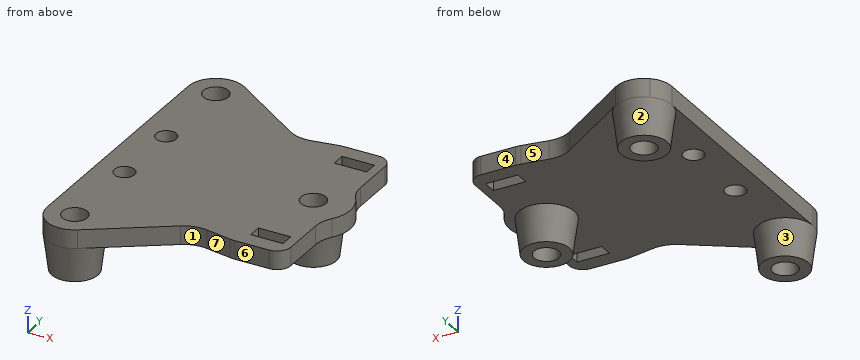
```python
from build123d import *

# Parameters (mm, degrees)
SKETCH_1_R          = 2.2
SKETCH_1_R_2        = 2.7
EXTRUDE_1_DEPTH     = 4
CUT_EXTRUDE_1_REACH = 59.017
EXTRUDE_START       = -4
SKETCH_6_W          = 7
SKETCH_6_H          = 3
SKETCH_6_R          = 2.7
EXTRUDE_3_DEPTH     = 4
FILLET_1_R          = 7
FILLET_2_R          = 3


with BuildPart() as part:
    # 草图1 → 凸台-拉伸1 (new body)
    with BuildSketch(Plane.XY):
        with BuildLine():
            Line((-22.03836949, 31.611607058), (-45, 12.5))
            Line((-45, 12.5), (-45, -12.5))
            Line((-45, -12.5), (-22.03836949, -31.611607058))
            ThreePointArc((-22.03836949, -31.611607058), (-18.500125226, -32.992489036), (-14.841614052, -31.972046241))
            Line((-14.841614052, -31.972046241), (22.677847931, -6.629394988))
            ThreePointArc((22.677847931, -6.629394988), (26.2, 0), (22.677847931, 6.629394988))
            Line((22.677847931, 6.629394988), (-14.841614052, 31.972046241))
            ThreePointArc((-14.841614052, 31.972046241), (-18.500125226, 32.992489036), (-22.03836949, 31.611607058))
        make_face()
        with Locations((-18.2, -8)):
            Circle(SKETCH_1_R, mode=Mode.SUBTRACT)
        with Locations((-18.2, 8)):
            Circle(SKETCH_1_R, mode=Mode.SUBTRACT)
        with Locations((-34.2, 0)):
            Circle(SKETCH_1_R, mode=Mode.SUBTRACT)
        with Locations((-18.2, 27)):
            Circle(SKETCH_1_R_2, mode=Mode.SUBTRACT)
        with Locations((-18.2, -27)):
            Circle(SKETCH_1_R_2, mode=Mode.SUBTRACT)
        with Locations((18.2, 0)):
            Circle(SKETCH_1_R_2, mode=Mode.SUBTRACT)
    extrude(amount=EXTRUDE_1_DEPTH)

    # 草图4 → 旋转1 (revolve)
    with BuildSketch(Plane(origin=(-25.021499827, 16.900859193, 0), x_dir=(0, 0, -1), z_dir=(0.8286743735186554, -0.5597309913462574, 0)), mode=Mode.PRIVATE) as revolve_1_sk:
        Polygon((7.7, 17.187104043), (7.7, 14.887104043), (0, 14.887104043), (0, 18.187104043), align=None)
    revolve_1 = revolve(revolve_1_sk.sketch.rotate(Axis((-18.2, 27, 1000.278995542), (0, 0, -1)), 55.962803956), axis=Axis((-18.2, 27, 1000.278995542), (0, 0, -1)))

    # 镜向1: 旋转1 across plane
    add(revolve_1.mirror(Plane.ZX))

    # 草图5 → 切除-拉伸1 (cut, up to next)
    with BuildSketch(Plane.XY.offset(4), mode=Mode.PRIVATE) as cut_extrude_1_sk1:
        with BuildLine():
            Line((-24.2, -27), (-24.2, 27))
            ThreePointArc((-24.2, 27), (-23.632780915, 29.546545018), (-22.03836949, 31.611607058))
            Line((-22.03836949, 31.611607058), (-45, 12.5))
            Line((-45, 12.5), (-45, -12.5))
            Line((-45, -12.5), (-22.03836949, -31.611607058))
            ThreePointArc((-22.03836949, -31.611607058), (-23.632780915, -29.546545018), (-24.2, -27))
        make_face()
    cut_extrude_1_tool1 = extrude(cut_extrude_1_sk1.sketch, amount=-CUT_EXTRUDE_1_REACH, mode=Mode.PRIVATE) & part.part
    add(cut_extrude_1_tool1.solids().sort_by_distance((-33.15819, 0, 4))[0], mode=Mode.SUBTRACT)

    # 草图6 → 凸台-拉伸3 (add)
    with BuildSketch(Plane.XY.offset(4).offset(EXTRUDE_START)):
        Polygon((12.5, -13.504057816), (3.649903477, -19.481886332), (12.5, -21), (23.5, -21), (23.5, 21), (12.5, 21), (3.649903477, 19.481886332), (12.5, 13.504057816), align=None)
        with Locations((18, -16)):
            Rectangle(SKETCH_6_W, SKETCH_6_H, mode=Mode.SUBTRACT)
        with Locations((18.2, 0)):
            Circle(SKETCH_6_R, mode=Mode.SUBTRACT)
        with Locations((18, 16)):
            Rectangle(SKETCH_6_W, SKETCH_6_H, mode=Mode.SUBTRACT)
    extrude(amount=EXTRUDE_3_DEPTH)

    # 圆角1
    fillet_1_edges = [part.edges().sort_by_distance(p)[0] for p in [
        (12.5, -21, 2),
        (3.649903477, -19.481886332, 2),
        (23.5, -5.992495307, 2),
        (23.5, 5.992495307, 2),
        (12.5, 21, 2),
        (3.649903477, 19.481886332, 2),
    ]]
    fillet(fillet_1_edges, radius=FILLET_1_R)

    # 圆角2
    fillet_2_edges = [part.edges().sort_by_distance(p)[0] for p in [
        (23.5, -21, 2),
        (23.5, 21, 2),
    ]]
    fillet(fillet_2_edges, radius=FILLET_2_R)

    # 草图7 → 旋转2 (revolve)
    with BuildSketch(Plane(origin=(6.459619467, 8.708524022, 0), x_dir=(0.8031661431318494, -0.5957551061692293, 0), z_dir=(0.5957551061692293, 0.8031661431318494, 0)), mode=Mode.PRIVATE) as revolve_2_sk:
        Polygon((11.917623805, 7.7), (11.917623805, 0), (8.617623805, 0), (9.617623805, 7.7), align=None)
    revolve(revolve_2_sk.sketch.rotate(Axis((18.2, 0, 0), (0, 0, -1)), 143.433519356), axis=Axis((18.2, 0, 0), (0, 0, -1)))


solid = part.part
```
Read the model definition and answer for the solid it produces. Units are mm, in the model's axes. Face numbers are marked on the shaded views. A direction names the side the tool comes from. Give positions to 0.01 mm unless a question says otherwise; leave off trailing zeros. Order: outer loops, then holes, each group sorted by start corner. A loop starts at its lowest first (then second) coordinate and runs counter-clockwise, first axis right, second up.
(1) Find section D-D (z = -5.25). Give the vertices of the cut face in (x, y).
(2) For the marked faces 5, 6 and 7, determine the directions among +Z, -Z, +X, -X, +Y, -Y from which every point of the face is accessible in a straight line to the end or side of a thin tool.
(3) Find section B-B (x = -18.2). Give the vertices of the cut face in (y, z).
(4) Find section A-A (y = -16.5). Give the vertices of the cut face in (x, z).
(5) Find section C-C (x = 18.2). Give the vertices of the cut face in (y, z), plus the area to 3 significant figures.
(6) For a pull along Y with two mould halves and no side action, classify the marked faces 1, 2, 3 and 4 as released by +Y, released by -Y, zero draft, split by the parting line, or undercut.
(7) Given pin 1 (3 mm diameter, centred on x = -15, y = 14, fed in from -Z); pin 2 (6 mm diameter, centred on x = 1.5, z = -2.5, fed in from -Y); pin 3 (1.2 mm diameter, centred on y = 11.5, z = 1.5, fed in from +X), each flat-ended and moving along its own axis, determine where each tip first touches the part or whether it passes through.
(8) Straight lines are drawn through the part: L1, parallel to Y at x = -18.2, z = 1.9; L2, parallel to X at y = -16, z = 1.75; L3, parallel to Z at x = -19, y = -13. For each, find the intervals that lie inside material, in ascending order.
Result sheet:
1. outline: circle Ø10.64 at (-18.2, -27); circle Ø10.64 at (-18.2, 27); circle Ø10.64 at (18.2, 0); hole circle Ø5.4 at (-18.2, -27); hole circle Ø5.4 at (-18.2, 27); hole circle Ø5.4 at (18.2, 0)
2. face 5: +Z, -Z, +Y
2. face 6: +Z, -Z, +X, -Y
2. face 7: +Z, -Z, -Y
3. outline: (-33, 0) - (-32, -7.7) - (-29.7, -7.7) - (-29.7, 4) - (-33, 4) - close; (-24.3, -7.7) - (-22, -7.7) - (-21, 0) - (-10.2, 0) - (-10.2, 4) - (-24.3, 4) - close; (-5.8, 0) - (5.8, 0) - (5.8, 4) - (-5.8, 4) - close; (10.2, 0) - (21, 0) - (22, -7.7) - (24.3, -7.7) - (24.3, 4) - (10.2, 4) - close; (29.7, -7.7) - (32, -7.7) - (33, 0) - (33, 4) - (29.7, 4) - close
4. outline: (-24.2, 0) - (14.5, 0) - (14.5, 4) - (-24.2, 4) - close; (21.5, 0) - (23.5, 0) - (23.5, 4) - (21.5, 4) - close
5. outline: (-21, 0) - (-17.5, 0) - (-17.5, 4) - (-21, 4) - close; (-14.5, 0) - (-6, 0) - (-5, -7.7) - (-2.7, -7.7) - (-2.7, 4) - (-14.5, 4) - close; (2.7, -7.7) - (5, -7.7) - (6, 0) - (14.5, 0) - (14.5, 4) - (2.7, 4) - close; (17.5, 0) - (21, 0) - (21, 4) - (17.5, 4) - close
5. area: 166 mm2
6. face 1: released by -Y
6. face 2: undercut
6. face 3: undercut
6. face 4: released by +Y
7. pin 1: stops at z = 0
7. pin 2: stops at y = -22.05
7. pin 3: stops at x = 23.5
8. L1: y = -33 to -29.7, -24.3 to -10.2, -5.8 to 5.8, 10.2 to 24.3, 29.7 to 33
8. L2: x = -24.2 to 14.5, 21.5 to 23.5
8. L3: z = 0 to 4
